from build123d import *

# Parameters (mm, degrees)
SCHIZZO1_R                    = 13.5
ESTRUSIONE_ESTRUSIONE1_DEPTH  = 8
SCHIZZO2_R                    = 10.5
TAGLIO_ESTRUSIONE1_DEPTH      = 7
SCHIZZO3_R                    = 7.5
TAGLIO_ESTRUSIONE2_DEPTH      = 2
TAGLIO_ESTRUSIONE4_DEPTH      = 14.5
TAGLIO_ESTRUSIONE4_DEPTH_BACK = 14.5


with BuildPart() as part:
    # Schizzo1 → Estrusione-Estrusione1 (new body)
    with BuildSketch(Plane(origin=(0, 0, 0), x_dir=(1, 0, 0), z_dir=(0, 1, 0))):
        Circle(SCHIZZO1_R)
    extrude(amount=ESTRUSIONE_ESTRUSIONE1_DEPTH)

    # Schizzo2 → Taglio-Estrusione1 (cut)
    with BuildSketch(Plane(origin=(0, 8, 0), x_dir=(1, 0, 0), z_dir=(0, 1, 0))):
        Circle(SCHIZZO2_R)
    extrude(amount=-TAGLIO_ESTRUSIONE1_DEPTH, mode=Mode.SUBTRACT)

    # Schizzo3 → Taglio-Estrusione2 (cut, through all)
    with BuildSketch(Plane(origin=(0, 1, 0), x_dir=(1, 0, 0), z_dir=(0, 1, 0))):
        Circle(SCHIZZO3_R)
    extrude(amount=-TAGLIO_ESTRUSIONE2_DEPTH, mode=Mode.SUBTRACT)

    # Schizzo4 → Taglio-Estrusione4 (cut, two sides)
    with BuildSketch(Plane(origin=(0, 0, 0), x_dir=(0, 0, -1), z_dir=(1, 0, 0))) as taglio_estrusione4_sk:
        with BuildLine():
            Line((2.140854023, 8), (-2.059200669, 8))
            Line((-2.059200669, 8), (-2.059200669, 4.1))
            ThreePointArc((-2.059200669, 4.1), (0.040826677, 1.999972654), (2.140854023, 4.1))
            Line((2.140854023, 4.1), (2.140854023, 8))
        make_face()
    extrude(amount=TAGLIO_ESTRUSIONE4_DEPTH, mode=Mode.SUBTRACT)
    extrude(taglio_estrusione4_sk.sketch, amount=-TAGLIO_ESTRUSIONE4_DEPTH_BACK, mode=Mode.SUBTRACT)


solid = part.part
Work out the finished part from the listing and answer in its coordinate system (mm). A direction names the side the tool comes from. Give positions to 0.01 mm unless a question says otherwise; leave off trailing zeros. Loops run counter-clockwise (first coordinate to the right, second up) from the corner with the lowest first, then second, coordinate; pieces in that order, holes last. Notation, with made-up numbers: (-39, 81.5) -> (-33, 81.5) arc R20 cw to (-33, 98.5) -> close; hole circle Ø3 at (69.5, 24). An arc over 180 degrees is marked (long way). Use a Markdown table: item, result. Add a question column.
1) Consider line 1 along X through (y, z) = (0.75, 0); line 2 along Z through (x, y) = (0, 1.25). Determine where each line is inside the solid, lowest interval first.
2) For a pull along X with two mould halves and no side action, classify faces 1 (the flat face through (0, 8, 11)), 2 (the cylindrical face through (12.47, 3.94, 5.17)), 3 (the cylindrical face through (10, 4.5, -3.2)), 4 (the cylindrical face through (-7.493, 0.507, -0.33)) as +X half, -X half, draft (parallel to the pull), parting line (faces both ways), or undercut.
3) The part is cut by section D-D, the plane z = -10. Determine the outline of the cut face in (x, y), plus the area to 3 significant figures.
4) The part is cut by section A-A, the plane x = 0. Determine the outline of the cut face in (y, z).
5) The part is cut by section C-C, the plane z = 6.5. Determine the outline of the cut face in (x, y), plus the area to 3 significant figures.
6) Each of these flat-tipped pins is pushed along its axis until it touches: P1, Ø2.5, axis at x = 11, y = 7, coming from the -Z side; P2, Ø4, axis at x = 2.5, y = 4.5, coming from the -Z side; P3, Ø2.5, axis at x = -12, y = 5.5, coming from the +Z side. Where does it stop, or does it pass through?
7) The part is cut by section B-B, the plane y = 6. Determine the outline of the cut face in (x, z), plus the area to 3 significant figures.
8) Which of the six approach directions +Z, -Z, +X, -X, +Y, -Y give full straight-line access (tool end or side, diameter ignored) to faces 5 (the flat face through (5, 1, 7)), 6 (the flat face through (6, 0, 6)), 7 (the flat face through (-12, 6, 2.059))?
Reported:
| question | item | result |
|---|---|---|
| 1 | line 1 | x = -13.5 to -7.5, 7.5 to 13.5 |
| 1 | line 2 | z = -13.5 to -10.5, 10.5 to 13.5 |
| 2 | face 1 | draft |
| 2 | face 2 | parting line |
| 2 | face 3 | undercut |
| 2 | face 4 | undercut |
| 3 | outline | (-9.07, 0) -> (9.07, 0) -> (9.07, 8) -> (3.2, 8) -> (3.2, 1) -> (-3.2, 1) -> (-3.2, 8) -> (-9.07, 8) -> close |
| 3 | area | 100 mm^2 |
| 4 | outline | (0, -13.5) -> (8, -13.5) -> (8, -10.5) -> (1, -10.5) -> (1, -7.5) -> (0, -7.5) -> close; (0, 7.5) -> (1, 7.5) -> (1, 10.5) -> (8, 10.5) -> (8, 13.5) -> (0, 13.5) -> close |
| 5 | outline | (-11.83, 0) -> (-3.74, 0) -> (-3.74, 1) -> (-8.25, 1) -> (-8.25, 8) -> (-11.83, 8) -> close; (3.74, 0) -> (11.83, 0) -> (11.83, 8) -> (8.25, 8) -> (8.25, 1) -> (3.74, 1) -> close |
| 5 | area | 66.4 mm^2 |
| 6 | P1 | stops at z = -9.34 |
| 6 | P2 | stops at z = -13.49 |
| 6 | P3 | stops at z = 8.17 |
| 7 | outline | (-13.34, 2.06) -> (-10.3, 2.06) arc R10.5 cw to (10.3, 2.06) -> (13.34, 2.06) arc R13.5 ccw to start; (-13.33, -2.14) arc R13.5 ccw to (13.33, -2.14) -> (10.28, -2.14) arc R10.5 cw to (-10.28, -2.14) -> close |
| 7 | area | 201 mm^2 |
| 8 | face 5 | +Y |
| 8 | face 6 | +Z, -Z, +X, -X, -Y |
| 8 | face 7 | +X, -X, +Y |
